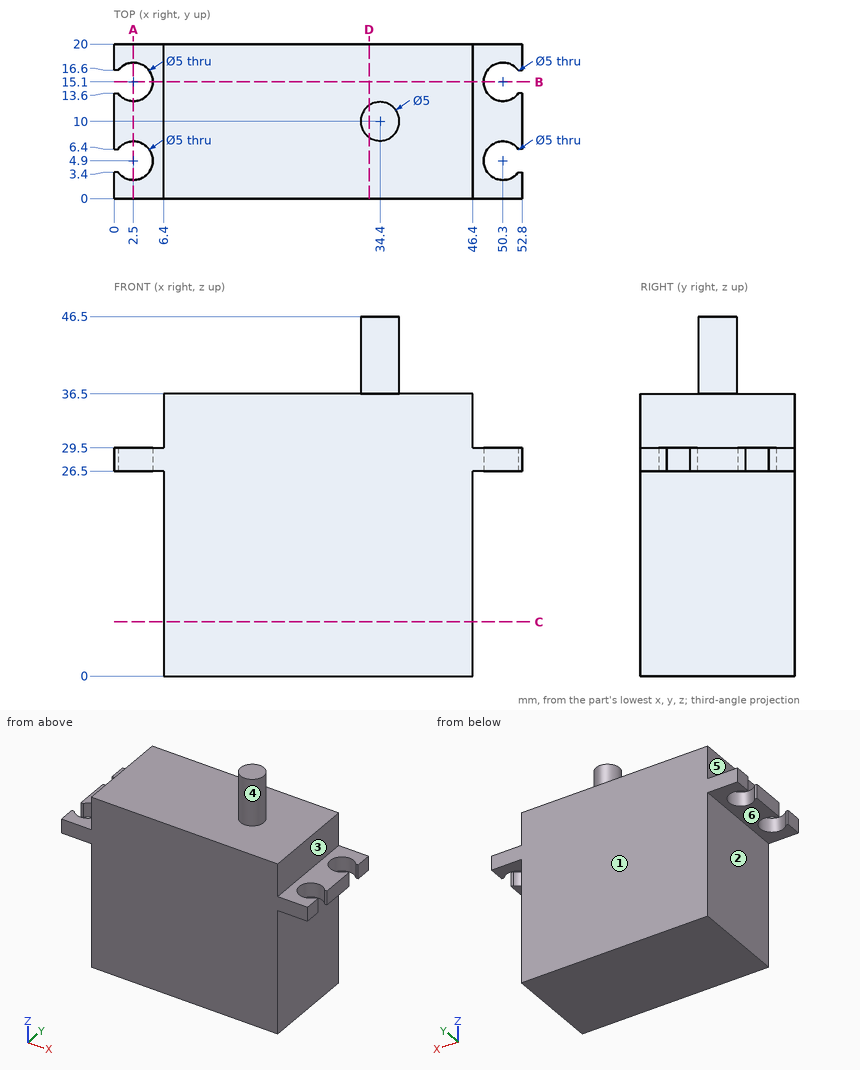
For this review, use the dimensioned drawing (mm, ordinates from the lowest corner) and the shaded views. A direction names the side the tool comes from. Coordinates: 2 decimals unless noted, no trailing zeros. Loops run counter-clockwise (first coordinate to the right, second up) from the corner with the lowest first, then second, coordinate; pieces in that order, holes last. Notation, with made-up numbers: (-23, 86) -> (17, 86) arc R31 ccw to (17, 123) -> close; hole circle Ø9 at (9, 80.25). An arc over 180 degrees is marked (long way). Use a Markdown table: item, result. Add a question column.
1. To check wall thickness, follow line 1 (Y direction, x = 50.3, z = 28.3); line 2 (Z direction, x = 33, y = 16); line 3 (Z direction, x = 47.5, y = 16.75). State the ranges of each line that lie inside material, in increasing order.
2. Machinability: for the marked faces 4, 5 and 6, which of the approach directions +Z, -Z, +X, -X, +Y, -Y give a long, thin tool a straight path to every point of the face, cutting with its end or side? Answer none if there is none.
3. Clearance check with flat-ended pins moving along their axes: pin 1 Ø6.5 at (x, y) = (2.5, 15.1) entering from -Z; pin 2 Ø10 at (x, y) = (26, 10) entering from +Z; pin 3 Ø2 at (y, z) = (10.5, 32.5) entering from +X. State where each tip first meets the part, or that it passes through.
4. Add section A-A on x = 2.5. Write out the cut boundary in (y, z), plus the area to 3 significant figures.
5. Add section D-D on x = 33. Write out the cut boundary in (y, z).
6. Add section B-B on y = 15.1. Write out the cut boundary in (x, z).
7. Draft analysis for pull direction X (two halves, no side actions). For the marked faces 1, 2 and 3, state which applies: pulls with the +X half, pulls with the -X half, needs draft (parallel to the pull), parting line crosses it, or undercut.
8. Add section C-C on z = 7. Write out the cut boundary in (x, y).
Returned:
| question | item | result |
|---|---|---|
| 1 | line 1 | y = 0 to 2.4, 7.4 to 12.6, 17.6 to 20 |
| 1 | line 2 | z = 0 to 36.5 |
| 1 | line 3 | z = 26.5 to 29.5 |
| 2 | face 4 | +Z |
| 2 | face 5 | +Z, -X, +Y, -Y |
| 2 | face 6 | -Z, -X, +Y, -Y |
| 3 | pin 1 | stops at z = 26.5 |
| 3 | pin 2 | stops at z = 36.5 |
| 3 | pin 3 | stops at x = 46.4 |
| 4 | outline | (0, 26.5) -> (2.4, 26.5) -> (2.4, 29.5) -> (0, 29.5) -> close; (7.4, 26.5) -> (12.6, 26.5) -> (12.6, 29.5) -> (7.4, 29.5) -> close; (17.6, 26.5) -> (20, 26.5) -> (20, 29.5) -> (17.6, 29.5) -> close |
| 4 | area | 30.0 mm² |
| 5 | outline | (0, 0) -> (20, 0) -> (20, 36.5) -> (12.07, 36.5) -> (12.07, 46.5) -> (7.93, 46.5) -> (7.93, 36.5) -> (0, 36.5) -> close |
| 6 | outline | (5, 26.5) -> (6.4, 26.5) -> (6.4, 0) -> (46.4, 0) -> (46.4, 26.5) -> (47.8, 26.5) -> (47.8, 29.5) -> (46.4, 29.5) -> (46.4, 36.5) -> (6.4, 36.5) -> (6.4, 29.5) -> (5, 29.5) -> close |
| 7 | face 1 | needs draft |
| 7 | face 2 | pulls with the -X half |
| 7 | face 3 | pulls with the +X half |
| 8 | outline | (6.4, 0) -> (46.4, 0) -> (46.4, 20) -> (6.4, 20) -> close |
